from build123d import *

# Parameters (mm, degrees)
F1_DEPTH = 1.5
F3_DEPTH = 6
F5_DEPTH = 3


with BuildPart() as f1:
    # F0 (on Top) → F1 (new body)
    with BuildSketch(Plane.XY):
        Polygon((16.25, 0), (0, 0), (-16.25, 0), (-16.25, -8.975), (16.25, -8.975), align=None)
        Polygon((-16.25, 0), (0, 0), (16.25, 0), (16.25, 8.975), (-16.25, 8.975), align=None)
        with BuildLine():
            Line((-16.25, -8.975), (-16.25, 0))
            Line((-16.25, 0), (-16.25, 8.975))
            ThreePointArc((-16.25, 8.975), (-25.225, 0), (-16.25, -8.975))
        make_face()
        with BuildLine():
            Line((16.25, 8.975), (16.25, 0))
            Line((16.25, 0), (16.25, -8.975))
            ThreePointArc((16.25, -8.975), (25.225, 0), (16.25, 8.975))
        make_face()
    extrude(amount=F1_DEPTH)

    # F2 (on face) → F3 (join)
    with BuildSketch(Plane.XY.offset(1.5)):
        Polygon((0, 8.975), (0, -0.99409), (0, -8.975), (12.25, -8.975), (12.25, 8.975), align=None)
        Polygon((0, -8.975), (0, -0.99409), (0, 8.975), (-12.25, 8.975), (-12.25, -8.975), align=None)
    extrude(amount=F3_DEPTH)

    # F4 (on face) → F5 (join)
    with BuildSketch(Plane.XY.offset(7.5)):
        Polygon((5.15, -6.175), (0, -6.175), (-5.15, -6.175), (-6.175, -5.15), (-6.175, -4.15), (-9.175, -4.15), (-9.175, -8.975), (9.175, -8.975), (9.175, -4.15), (6.175, -4.15), (6.175, -5.15), align=None)
        Polygon((-5.15, 6.175), (0, 6.175), (5.15, 6.175), (6.175, 5.15), (6.175, 4.15), (9.175, 4.15), (9.175, 8.975), (-9.175, 8.975), (-9.175, 4.15), (-6.175, 4.15), (-6.175, 5.15), align=None)
    extrude(amount=F5_DEPTH)


solid = f1.part
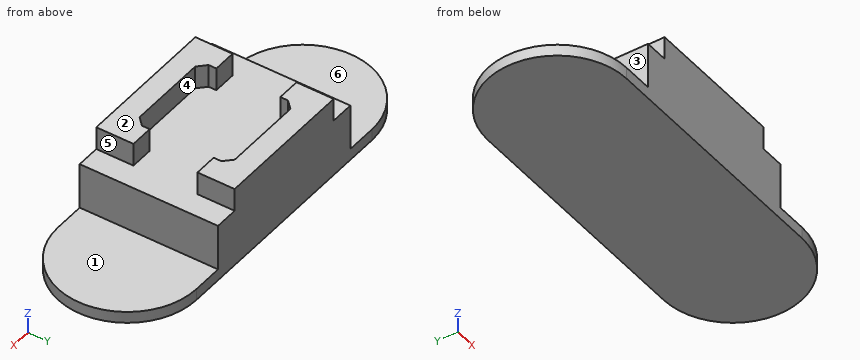
Work out the finished part from the listing and answer in its coordinate system (mm). Face numbers are marked on the shaded views. A direction names the side the tool comes from. Give positions to 0.01 mm unless a question says otherwise; leave off trailing zeros. Loops run counter-clockwise (first coordinate to the right, second up) from the corner with the lowest first, then second, coordinate; pieces in that order, holes last. Notation, with made-up numbers: (-6, 12) -> (13, 12) arc R10 cw to (13, 30) -> close; hole circle Ø1 at (37, 6.25). An arc over 180 degrees is marked (long way). Use a Markdown table: item, result. Add a question column.
1. Section B-B on y = 0 is taken. Determine the outline of the cut face in (x, z) (3 decimals).
2. Determine the mould class of the marked faces 3, 4, 5 and 6 for opening direction X: released by +X, released by -X, zero draft, split by the parting line, or undercut.
3. Section C-C on z = 3.5 is taken. Determine the outline of the cut face in (x, y) (3 decimals), and give its area (3 significant figures).
4. Section A-A on z = 9.25 is taken. Determine the outline of the cut face in (x, y) (3 decimals).
5. Section D-D on x = 18 is taken. Determine the outline of the cut face in (y, z), and give its area (3 significant figures).
6. For the marked faces 1 and 2, determine the directions among +Z, -Z, +X, -X, +Y, -Y from which every point of the face is accessible in a straight line to the end or side of a thin tool.
7. Find the intervals of material crossed by probe 1 along Y at (x, z) = (-1.5, 9.75) (3 decimals); probe 2 along Y at (x, z) = (-8.5, 8.5) (3 decimals); probe 3 along Z at (x, y) = (-10.5, -8), in increasing order.
8. Flat-ended cylindrical pins translate along their axes: pin 1 Ø10.5 at (x, y) = (19.5, -3) entering from +Z; pin 2 Ø1 at (x, y) = (-16.5, 4) entering from -Z; pin 3 Ø0.5 at (y, z) = (4.5, 8.5) entering from -X (3 decimals); pin 4 Ø1.8 at (y, z) = (-3, 3.5) entering from +X. Find the tip coordinate at first contact, or state that the pin passes through.
Results below:
| question | item | result |
|---|---|---|
| 1 | outline | (-25.225, 0) -> (25.225, 0) -> (25.225, 1.5) -> (12.25, 1.5) -> (12.25, 7.5) -> (-12.25, 7.5) -> (-12.25, 1.5) -> (-25.225, 1.5) -> close |
| 2 | face 3 | released by -X |
| 2 | face 4 | undercut |
| 2 | face 5 | released by +X |
| 2 | face 6 | zero draft |
| 3 | outline | (-12.25, -8.975) -> (12.25, -8.975) -> (12.25, 8.975) -> (-12.25, 8.975) -> close |
| 3 | area | 440 mm^2 |
| 4 | outline | (-9.175, -8.975) -> (9.175, -8.975) -> (9.175, -4.15) -> (6.175, -4.15) -> (6.175, -5.15) -> (5.15, -6.175) -> (-5.15, -6.175) -> (-6.175, -5.15) -> (-6.175, -4.15) -> (-9.175, -4.15) -> close; (-9.175, 4.15) -> (-6.175, 4.15) -> (-6.175, 5.15) -> (-5.15, 6.175) -> (5.15, 6.175) -> (6.175, 5.15) -> (6.175, 4.15) -> (9.175, 4.15) -> (9.175, 8.975) -> (-9.175, 8.975) -> close |
| 5 | outline | (-8.8, 0) -> (8.8, 0) -> (8.8, 1.5) -> (-8.8, 1.5) -> close |
| 5 | area | 26.4 mm^2 |
| 6 | face 1 | +Z, +X, +Y, -Y |
| 6 | face 2 | +Z, +X, -X, +Y, -Y |
| 7 | probe 1 | y = -8.975 to -6.175, 6.175 to 8.975 |
| 7 | probe 2 | y = -8.975 to -4.15, 4.15 to 8.975 |
| 7 | probe 3 | z = 0 to 7.5 |
| 8 | pin 1 | stops at z = 1.5 |
| 8 | pin 2 | stops at z = 0 |
| 8 | pin 3 | stops at x = -9.175 |
| 8 | pin 4 | stops at x = 12.25 |
